Verification items for the finished model (mm, model axes). Face numbers are marked on the shaded views. Round coordinates to 2 decimals unless told otherwise and drop trailing zeros. Order: outer loops, then holes, each group sorted by start corner. A loop starts at its lowest first (then second) coordinate and runs counter-clockwise, first axis right, second up. Notation, with made-up numbers: M 70,29.5 L 110,29.5 A12 ccw 110,51.5 Z; hole C -36.75,43 d5. An arc over 180 degrees is marked long. Use one line per item in the form item = value. Start each with the question number.
Item 1: Go/stop test with flat-tipped pins: pin 1 Ø4 at (y, z) = (58.5, -17.5) entering from -X; pin 2 Ø3 at (x, z) = (23, -38) entering from +Y; pin 3 Ø1.5 at (x, z) = (27.5, -32.5) entering from +Y. Record where each tip stops, or that it passes through.
Item 2: Thickness scan on probe 1 along Y at (x, z) = (36, -16.5); probe 2 along Y at (x, z) = (21.5, -10); probe 3 along X at (y, z) = (51.5, -38). Record the ranges inside material, lowest first. Write a range as [from, to].
Item 3: Cross-section at C-C on z = -3. Enter the section's corners in (x, y), then the cut area to 3 significant figures.
Item 4: Cross-section at B-B on y = 20. Enter the section's corners in (x, z), then the cut area to 3 significant figures.
Item 5: Release check for a two-part mould opening along Y. For the marked faces 1, 2 and 3 record: +Y half, -Y half, draft (parallel to the pull), parting line (faces both ways), or undercut.
Item 6: Cross-section at A-A on z = -12. Enter the section's corners in (x, y).
from build123d import *

# Parameters (mm, degrees)
F0_R     = 18
F0_R_2   = 10.5
F1_DEPTH = 50
F2_R     = 8.5
F3_R     = 8.5


with BuildPart() as f1:
    # F0 (on Top) → F1 (new body)
    with BuildSketch(Plane.XY):
        Polygon((0, 44), (0, 0), (120, 0), (117.837585, 43.946831), (76, 76), (32, 76), align=None)
        with Locations((36, 36)):
            Circle(F0_R, mode=Mode.SUBTRACT)
        with Locations((84, 20)):
            Circle(F0_R_2, mode=Mode.SUBTRACT)
    extrude(amount=-F1_DEPTH)

    # F2
    f2_edges = [f1.edges().sort_by_distance(p)[0] for p in [
        (96.918792, 59.973416, 0),
        (96.918792, 59.973416, -50),
    ]]
    fillet(f2_edges, radius=F2_R)

    # F3
    f3_edges = [f1.edges().sort_by_distance(p)[0] for p in [
        (16, 60, 0),
        (16, 60, -50),
    ]]
    fillet(f3_edges, radius=F3_R)


solid = f1.part
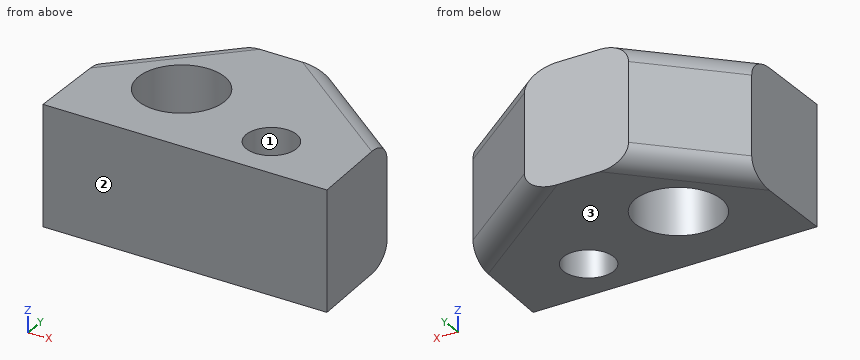
Output values:
q1.pin_1 = 12.5
q1.pin_2 = 68.5
q1.pin_3 = 72.25
q2.probe_1 = [0, 18], [54, 76]
q2.probe_2 = [0, 25.33], [46.67, 65.5]
q2.probe_3 = [7.5, 26.85], [45.15, 107.98]
q3.outline = M 0,0 L 120,0 L 117.97,41.3 L 72.68,76 L 34.86,76 L 0,41.14 Z; hole C 36,36 d36; hole C 84,20 d21
q3.area = 6,250 mm2
q4.outline = M 0,-50 L 27.75,-50 L 27.75,0 L 0,0 Z; M 44.25,-50 L 73.5,-50 L 73.5,0 L 44.25,0 Z; M 94.5,-50 L 119.02,-50 L 119.02,0 L 94.5,0 Z
q4.area = 4,080 mm2
q5.face_1 = undercut
q5.face_2 = -Y half
q5.face_3 = draft
q6.outline = M 0,0 L 120,0 L 117.84,43.95 L 76,76 L 32,76 L 0,44 Z; hole C 36,36 d36; hole C 84,20 d21
